Source: CAD feature listing. Evaluate the final solid. Frame: model axes, mm. A direction names the side the tool comes from. Give positions to 0.01 mm unless a question says otherwise; leave off trailing zeros. Write each loop counter-clockwise with the first axis right and the second up, starting at its lowest first coordinate (ties: lowest second). Pieces come first, ordered by that corner, then holes. Notation, with made-up numbers: (38, 19) -> (88, 19) arc R21 cw to (88, 52) -> close; hole circle Ø6 at (69.5, -18.75). An arc over 180 degrees is marked (long way). Use one line per item in the form item = value. Start each with the question number.
(1) Set-up query: faces 4 (the face through (0.526, -1.729, 146.669)), 5 (the face through (-2, -0.25, 25)). Return all of +Z, -Z, +X, -X, +Y, -Y with unobstructed straight access to the full face (end or side cutting, diameter ignored); none if empty.
(2) Draft query along X for faces 1 (the face through (0.9, 1.52, 147.86)), 2 (the face through (0, 3.25, 74)), 3 (the face through (-0.67, -1.729, 46.617)). Return one class per face: pulls with the +X half, pulls with the -X half, needs draft (parallel to the pull), parting line crosses it, or undercut.
(3) Material intervals for line 1 along X through (y, z) = (-1.1, 85); line 2 along X through (y, z) = (0.95, 145); line 3 along Y through (x, z) = (3.5, 15), sorted ascending. Write a range as from..to.
(4) Cut plane A-A, the plane z = 65. Output: boundary loops of the cut face in (x, y).
(5) Cut plane B-B, the plane y = -1.5. Count the separate pieces of the cut face and the enclosed holes in it, and give its area (3 significant figures).
(6) First-contact query: P1, Ø1.8, axis at x = -0.5, z = 24.5, coming from the +Y side; P2, Ø4, axis at x = 0, z = 65, coming from the +Y side. Flat tips, straight axial feed; report the tip coordinate or a pass-through.
(7) Cut plane C-C, the plane z = 34. Output: boundary loops of the cut face in (x, y).
from build123d import *

# Parameters (mm, degrees)
EXTRUDE1_DEPTH  = 150
SKETCH2_R       = 3
EXTRUDE2_DEPTH  = 3.5
SKETCH_R        = 1.75
EXTRUDE3_DEPTH  = 151.208188858
LPATTERN1_COUNT = 40
LPATTERN1_PITCH = 20


with BuildPart() as part:
    # Sketch1 → Extrude1 (new body)
    with BuildSketch(Plane.XY):
        with BuildLine():
            Line((-4.5, -3.25), (4.5, -3.25))
            Line((4.5, -3.25), (4.5, 0.45))
            ThreePointArc((4.5, 0.45), (3.887627564, 0.659430585), (3.531754163, 1.2))
            Line((3.531754163, 1.2), (3.4, 1.2))
            Line((3.4, 1.2), (3.4, 1.7))
            Line((3.4, 1.7), (3.531754163, 1.7))
            ThreePointArc((3.531754163, 1.7), (3.887627564, 2.240569415), (4.5, 2.45))
            Line((4.5, 2.45), (4.5, 3.25))
            Line((4.5, 3.25), (-4.5, 3.25))
            Line((-4.5, 3.25), (-4.5, 2.45))
            ThreePointArc((-4.5, 2.45), (-3.887627564, 2.240569415), (-3.531754163, 1.7))
            Line((-3.531754163, 1.7), (-3.4, 1.7))
            Line((-3.4, 1.7), (-3.4, 1.2))
            Line((-3.4, 1.2), (-3.531754163, 1.2))
            ThreePointArc((-3.531754163, 1.2), (-3.887627564, 0.659430585), (-4.5, 0.45))
            Line((-4.5, 0.45), (-4.5, -3.25))
        make_face()
    extrude(amount=EXTRUDE1_DEPTH)

    # Sketch2 → Extrude2 (cut)
    with BuildSketch(Plane(origin=(0, 3.25, 0), x_dir=(1, 0, 0), z_dir=(0, 1, 0))):
        with Locations(Location((0, -5, 0), (0, 0, 270))):
            Circle(SKETCH2_R)
    extrude2 = extrude(amount=-EXTRUDE2_DEPTH, mode=Mode.SUBTRACT)

    # Sketch → Extrude3 (cut, through all)
    with BuildSketch(Plane(origin=(0, 3.25, 0), x_dir=(1, 0, 0), z_dir=(0, 1, 0))):
        with Locations(Location((0, -5, 0), (0, 0, 270))):
            Circle(SKETCH_R)
    extrude3 = extrude(amount=-EXTRUDE3_DEPTH, mode=Mode.SUBTRACT)

    # LPattern1: Extrude2, Extrude3 ×40
    with Locations(*[(0, 0, i * LPATTERN1_PITCH) for i in range(1, LPATTERN1_COUNT)]):
        add(extrude2, mode=Mode.SUBTRACT)
        add(extrude3, mode=Mode.SUBTRACT)


solid = part.part
Geometry says:
q1.face_4 = +Y, -Y
q1.face_5 = +Y
q2.face_1 = undercut
q2.face_2 = needs draft
q2.face_3 = undercut
q3.line_1 = -4.5..-1.75, 1.75..4.5
q3.line_2 = -3.63..-3, 3..3.63
q3.line_3 = -3.25..1.2, 1.7..3.25
q4.outline = (-4.5, -3.25) -> (-1.75, -3.25) -> (-1.75, -0.25) -> (-3, -0.25) -> (-3, 3.25) -> (-4.5, 3.25) -> (-4.5, 2.45) arc R1 cw to (-3.53, 1.7) -> (-3.4, 1.7) -> (-3.4, 1.2) -> (-3.53, 1.2) arc R1 cw to (-4.5, 0.45) -> close; (1.75, -3.25) -> (4.5, -3.25) -> (4.5, 0.45) arc R1 cw to (3.53, 1.2) -> (3.4, 1.2) -> (3.4, 1.7) -> (3.53, 1.7) arc R1 cw to (4.5, 2.45) -> (4.5, 3.25) -> (3, 3.25) -> (3, -0.25) -> (1.75, -0.25) -> close
q5.separate_pieces = 1
q5.enclosed_holes = 8
q5.area = 1,270 mm^2
q6.P1 = through
q6.P2 = -0.25
q7.outline = (-4.5, -3.25) -> (4.5, -3.25) -> (4.5, 0.45) arc R1 cw to (3.53, 1.2) -> (3.4, 1.2) -> (3.4, 1.7) -> (3.53, 1.7) arc R1 cw to (4.5, 2.45) -> (4.5, 3.25) -> (-4.5, 3.25) -> (-4.5, 2.45) arc R1 cw to (-3.53, 1.7) -> (-3.4, 1.7) -> (-3.4, 1.2) -> (-3.53, 1.2) arc R1 cw to (-4.5, 0.45) -> close
